Geometry: final body of the model. Coordinates: model frame, mm. A direction names the side the tool comes from. Give positions to 0.01 mm unless a question says otherwise; leave off trailing zeros. Write each loop counter-clockwise with the first axis right and the second up, starting at its lowest first coordinate (ties: lowest second). Pieces come first, ordered by that corner, then holes.
Q1. Cut plane C-C on z = 7. Return the cut outline in (x, y), plus the area to 3 significant figures.
Q2. Cut plane A-A on x = 0. Return the cut outline in (y, z), plus the area to 3 significant figures.
Q3. Line query: L1, parallel to Z at x = 0, y = 3.75; L2, parallel to Z at x = 0, y = 2; L3, parallel to Y at x = 1.25, z = 1.75. Output: solid intervals per line, ascending.
Q4. Pin query (flat end, axial travel): pin 1 (10 mm diameter, centred on x = 6.5, z = 0.5, fed in from -Y); pin 2 (1.5 mm diameter, centred on x = -3, y = 5.5, fed in from +Z); pin 3 (0.9 mm diameter, centred on x = 1, y = 7, fed in from -Z); pin 4 (3.5 mm diameter, centred on x = -7, z = -1, fed in from +Y). Return the tip coordinate at first contact, or that it passes through.
Q5. Draft query along X for faces 4 (the face through (-6, 6, 0)), 5 (the face through (2, 0, 0)), 6 (the face through (-7.784, 7.014, -4.078)), 7 (the face through (-2.17, 3.94, 9.76)). Return one class per face: pulls with the +X half, pulls with the -X half, needs draft (parallel to the pull), parting line crosses it, or undercut.
Q6. Cut plane D-D on y = 4. Return the cut outline in (x, z), plus the area to 3 significant figures.
Q7. Reachability of faces 1 (the face through (0, 5, -3)), 2 (the face through (0.35, 3.18, 8.56)), 3 (the face through (7.784, 7.014, 4.078)) from +Z, -Z, +X, -X, +Y, -Y: full face, straight path, thin tool, end or side. Return the list, or none.
Q8. Cut plane B-B on y = 7.75. Return the cut outline in (x, z), plus the area to 3 significant figures.
```python
from build123d import *

# Parameters (mm, degrees)
SKETCH1_R                                           = 10
BOSS_EXTRUDE1_DEPTH                                 = 6
CUT_EXTRUDE4_DEPTH                                  = 2.5
SKETCH9_R                                           = 10
BOSS_EXTRUDE2_DEPTH                                 = 2
CSK_FOR_M3_COUNTERSUNK_FLAT_HEAD_SCREW2_D           = 3.2
CSK_FOR_M3_COUNTERSUNK_FLAT_HEAD_SCREW2_CSINK_D     = 6.3
CSK_FOR_M3_COUNTERSUNK_FLAT_HEAD_SCREW2_CSINK_ANGLE = 90
CUT_EXTRUDE6_DEPTH                                  = 2
SKETCH18_R                                          = 1.7
CUT_EXTRUDE8_DEPTH                                  = 9


with BuildPart() as part:
    # Sketch1 → Boss-Extrude1 (new body)
    with BuildSketch(Plane(origin=(0, 0, 0), x_dir=(1, 0, 0), z_dir=(0, 1, 0))):
        Circle(SKETCH1_R)
    extrude(amount=BOSS_EXTRUDE1_DEPTH)

    # Sketch8 → Cut-Extrude4 (cut)
    with BuildSketch(Plane(origin=(0, 6, 0), x_dir=(1, 0, 0), z_dir=(0, 1, 0))):
        Polygon((3.464101615, 0), (1.732050808, 3), (-1.732050808, 3), (-3.464101615, 0), (-1.732050808, -3), (1.732050808, -3), align=None)
    extrude(amount=-CUT_EXTRUDE4_DEPTH, mode=Mode.SUBTRACT)

    # Sketch9 → Boss-Extrude2 (add)
    with BuildSketch(Plane(origin=(0, 6, 0), x_dir=(1, 0, 0), z_dir=(0, 1, 0))):
        Circle(SKETCH9_R)
    extrude(amount=BOSS_EXTRUDE2_DEPTH)

    # CSK for M3 Countersunk Flat Head Screw2 (through all)
    with Locations(Plane(origin=(0, 8, 0), x_dir=(1, 0, 0), z_dir=(0, 1, 0))):
        with Locations((0, 7), (0, -7)):
            CounterSinkHole(CSK_FOR_M3_COUNTERSUNK_FLAT_HEAD_SCREW2_D / 2, CSK_FOR_M3_COUNTERSUNK_FLAT_HEAD_SCREW2_CSINK_D / 2, counter_sink_angle=CSK_FOR_M3_COUNTERSUNK_FLAT_HEAD_SCREW2_CSINK_ANGLE)

    # Sketch16 → Cut-Extrude6 (cut)
    with BuildSketch(Plane(origin=(0, 8, 0), x_dir=(1, 0, 0), z_dir=(0, 1, 0))):
        Polygon((-6.426401471, 6.555437753), (-9.18, 1.53), (-9.18, -1.53), (-6.426401471, -6.555437753), (-1.53, -1.53), (1.53, -1.53), (6.426401471, -6.555437753), (9.18, -1.53), (9.18, 1.53), (6.426401471, 6.555437753), (1.53, 1.53), (-1.53, 1.53), align=None)
    extrude(amount=-CUT_EXTRUDE6_DEPTH, mode=Mode.SUBTRACT)

    # Sketch18 → Cut-Extrude8 (cut)
    with BuildSketch(Plane(origin=(0, 8, 0), x_dir=(1, 0, 0), z_dir=(0, 1, 0))):
        Circle(SKETCH18_R)
    extrude(amount=-CUT_EXTRUDE8_DEPTH, mode=Mode.SUBTRACT)


solid = part.part
```
Data:
1. outline: (-7.14, 0) - (-1.6, 0) - (-1.6, 6.45) - (-3.15, 8) - (-7.14, 8) - close; (1.6, 0) - (7.14, 0) - (7.14, 8) - (3.15, 8) - (1.6, 6.45) - close
1. area: 86.3 mm2
2. outline: (0, -10) - (7.85, -10) - (6.45, -8.6) - (0, -8.6) - close; (0, -5.4) - (6.45, -5.4) - (8, -3.85) - (8, -1.7) - (6, -1.7) - (6, -3) - (3.5, -3) - (3.5, -1.7) - (0, -1.7) - close; (0, 1.7) - (3.5, 1.7) - (3.5, 3) - (6, 3) - (6, 1.7) - (8, 1.7) - (8, 3.85) - (6.45, 5.4) - (0, 5.4) - close; (0, 8.6) - (6.45, 8.6) - (7.85, 10) - (0, 10) - close
2. area: 70.3 mm2
3. L1: z = -10 to -8.6, -5.4 to -3, 3 to 5.4, 8.6 to 10
3. L2: z = -10 to -8.6, -5.4 to -1.7, 1.7 to 5.4, 8.6 to 10
3. L3: y = 0 to 3.5, 6 to 8
4. pin 1: stops at y = 0
4. pin 2: stops at z = 9.74
4. pin 3: stops at z = -9.98
4. pin 4: stops at y = 6
5. face 4: undercut
5. face 5: needs draft
5. face 6: undercut
5. face 7: parting line crosses it
6. outline: circle Ø20 at (0, 0); hole (-3.46, 0) - (-1.73, -3) - (1.73, -3) - (3.46, 0) - (1.73, 3) - (-1.73, 3) - close; hole circle Ø3.2 at (0, -7); hole circle Ø3.2 at (0, 7)
6. area: 267 mm2
7. face 1: none
7. face 2: +Y, -Y
7. face 3: +Y
8. outline: circle Ø20 at (0, 0); hole (-9.18, -1.53) - (-6.43, -6.56) - (-1.53, -1.53) - (-0.74, -1.53) arc R1.7 ccw to (0.74, -1.53) - (1.53, -1.53) - (6.43, -6.56) - (9.18, -1.53) - (9.18, 1.53) - (6.43, 6.56) - (1.53, 1.53) - (0.74, 1.53) arc R1.7 ccw to (-0.74, 1.53) - (-1.53, 1.53) - (-6.43, 6.56) - (-9.18, 1.53) - close; hole circle Ø5.8 at (0, -7); hole circle Ø5.8 at (0, 7)
8. area: 128 mm2
